Read the model definition and answer for the solid it produces. Units are mm, in the model's axes. A direction names the side the tool comes from. Coordinates: 2 decimals unless noted, no trailing zeros. Loops run counter-clockwise (first coordinate to the right, second up) from the corner with the lowest first, then second, coordinate; pieces in that order, holes last. Notation, with made-up numbers: (20, 43) -> (62, 43) arc R11 cw to (62, 64) -> close; hole circle Ø11 at (69.5, -27.75). An arc over 180 degrees is marked (long way). Answer as a JSON object with one key per item and string values. Group by question number.
Q1. Straight lines are drawn through the part: line 1 along X through (y, z) = (3.25, 0); line 2 along Y through (x, z) = (4.25, 2.25); line 3 along Z through (x, y) = (-1, 1.75). For each, find the intervals that lie inside material, in ascending order. Write a range as [from, to].
Q2. The part is cut by section B-B on z = 0. Write down the section's boundary in (x, y).
Q3. Each of these flat-tipped pins is pushed along its axis until it touches: P1, Ø0.7, axis at x = -5, z = -0.5, coming from the -Y side; P2, Ø3.5, axis at x = 0, z = 0, coming from the -Y side; P3, Ø1.5, axis at x = 3, y = 8.5, coming from the -Z side; P4, Ø3, axis at y = 2, z = 3, coming from the -X side. Where does it stop, or does it pass through?
Q4. Determine the mould class of faces 1 (the flat face through (-0.8, 5, 4.8)), 2 (the flat face through (3.665, 7.292, -3.143)), 3 (the cylindrical face through (-4.446, 2.465, 0.697)) for opening direction Z: released by +Z, released by -Z, zero draft, split by the parting line, or undercut.
Q5. The part is cut by section C-C on x = -3.25. Write down the section's boundary in (y, z).
Q6. For faces 4 (the flat face through (2.2, 5, -4.3)), 5 (the flat face through (-3.143, 7.292, -3.665)), 6 (the cylindrical face through (4.006, 2.465, 2.049)), determine the directions among +Z, -Z, +X, -X, +Y, -Y from which every point of the face is accessible in a straight line to the end or side of a thin tool.
Q7. The part is cut by section A-A on x = 0. Write down the section's boundary in (y, z).
from build123d import *

# Parameters (mm, degrees)
SKETCH_1_R               = 4.5
EXTRUDE_1_DEPTH          = 10
SKETCH_2_R               = 5.25
EXTRUDE_2_DEPTH          = 5
CUT_EXTRUDE_3_DEPTH      = 10
PATTERN_CIRCULAR_2_COUNT = 20
SKETCH_5_R               = 1.5
CUT_EXTRUDE_4_DEPTH      = 10


with BuildPart() as part:
    # 스케치1 → 보스-돌출1 (new body)
    with BuildSketch(Plane(origin=(0, 0, 0), x_dir=(1, 0, 0), z_dir=(0, 1, 0))):
        with Locations(Location((0, 0, 0), (0, 0, 270))):
            Circle(SKETCH_1_R)
    extrude(amount=EXTRUDE_1_DEPTH)

    # 스케치2 → 보스-돌출2 (add)
    with BuildSketch(Plane(origin=(0, 10, 0), x_dir=(1, 0, 0), z_dir=(0, 1, 0))):
        with Locations(Location((0, 0, 0), (0, 0, 270))):
            Circle(SKETCH_2_R)
    extrude(amount=-EXTRUDE_2_DEPTH)

    # 스케치4 → 컷-돌출3 (cut)
    with BuildSketch(Plane(origin=(0, 10, 0), x_dir=(1, 0, 0), z_dir=(0, 1, 0))):
        Polygon((0, 4.4), (0.15, 4.4), (0.727350269, 5.4), (-0.727350269, 5.4), (-0.15, 4.4), align=None)
    cut_extrude_3 = extrude(amount=-CUT_EXTRUDE_3_DEPTH, mode=Mode.SUBTRACT)

    # 원형 패턴2: 컷-돌출3 ×20 about axis
    pattern_circular_2_axis = Axis((0, 0, 0), (0, 1, 0))
    for i in range(1, PATTERN_CIRCULAR_2_COUNT):
        add(cut_extrude_3.rotate(pattern_circular_2_axis, i * 360 / PATTERN_CIRCULAR_2_COUNT), mode=Mode.SUBTRACT)

    # 스케치5 → 컷-돌출4 (cut)
    with BuildSketch(Plane(origin=(0, 10, 0), x_dir=(1, 0, 0), z_dir=(0, 1, 0))):
        with Locations(Location((0, 0, 0), (0, 0, 270))):
            Circle(SKETCH_5_R)
    extrude(amount=-CUT_EXTRUDE_4_DEPTH, mode=Mode.SUBTRACT)


solid = part.part
Final values:
{
 "1": {"line 1": "x = [-4.4, -1.5], [1.5, 4.4]", "line 2": "y = [5, 10]", "line 3": "z = [-4.39, -1.12], [1.12, 4.39]"},
 "2": {"outline": "(-4.4, 0) -> (-1.5, 0) -> (-1.5, 10) -> (-4.4, 10) -> close; (1.5, 0) -> (4.4, 0) -> (4.4, 10) -> (1.5, 10) -> close"},
 "3": {"P1": "stops at y = 5", "P2": "stops at y = 0", "P3": "stops at z = -4.74", "P4": "stops at x = -4.21"},
 "4": {"face 1": "zero draft", "face 2": "undercut", "face 3": "released by +Z"},
 "5": {"outline": "(0, -3.11) -> (5, -3.11) -> (5, -3.71) -> (10, -3.71) -> (10, 3.71) -> (5, 3.71) -> (5, 3.11) -> (0, 3.11) -> close"},
 "6": {"face 4": "-Z, +X, -Y", "face 5": "-Z, +Y, -Y", "face 6": "+Z, +X, -Y"},
 "7": {"outline": "(0, -4.4) -> (10, -4.4) -> (10, -1.5) -> (0, -1.5) -> close; (0, 1.5) -> (10, 1.5) -> (10, 4.4) -> (0, 4.4) -> close"}
}
